The model under review builds one solid part; all positions refer to its coordinate system, in mm. A direction names the side the tool comes from. Coordinates: 2 decimals unless noted, no trailing zeros. Write each loop counter-clockwise with the first axis right and the second up, starting at its lowest first coordinate (ties: lowest second). Pieces come first, ordered by that corner, then holes. Notation, with made-up numbers: (-18.5, 6.5) - (38.5, 6.5) arc R11 ccw to (38.5, 10.5) - close; hole circle Ø10 at (10, 47.25). An arc over 180 degrees is marked (long way). Put each result on its own line as item: value.
from build123d import *

# Parameters (mm, degrees)
SKETCH_2_R          = 2.1
CUT_EXTRUDE_1_DEPTH = 50.216460661
CHAMFER_1_SIZE      = 0.5
CHAMFER_2_SIZE      = 0.5


with BuildPart() as part:
    # Эскиз1 → Повернуть1 (revolve)
    with BuildSketch(Plane.XY, mode=Mode.PRIVATE) as revolve_1_sk:
        Polygon((-22.5, 5), (-22.5, 2), (-20.5, 0), (-15.5, 0), (-15.5, 1.5), (-17.5, 1.5), (-17.5, 19.5), (-18.5, 19.5), (-18.5, 21.1), (-17.5, 21.1), (-17.5, 22.6), (-20, 22.6), (-21, 21.6), (-21, 13), (-32.5, 13), (-32.5, 5), align=None)
    revolve(revolve_1_sk.sketch.rotate(Axis((0, 0, 0), (0, 1, 0)), 270), axis=Axis((0, 0, 0), (0, 1, 0)))

    # Эскиз2 → Вырез-Вытянуть1 (cut, through all)
    with BuildSketch(Plane.XZ.offset(-5)):
        with Locations((0, 27.5)):
            Circle(SKETCH_2_R)
        with Locations((27.5, 0)):
            Circle(SKETCH_2_R)
        with Locations((0, -27.5)):
            Circle(SKETCH_2_R)
        with Locations((-27.5, 0)):
            Circle(SKETCH_2_R)
    extrude(amount=-CUT_EXTRUDE_1_DEPTH, mode=Mode.SUBTRACT)

    # Фаска1
    chamfer_1_edges = [part.edges().sort_by_distance(p)[0] for p in [
        (0, 0, 15.5),
        (0, 1.5, 15.5),
        (0, 22.6, 17.5),
    ]]
    chamfer(chamfer_1_edges, length=CHAMFER_1_SIZE)

    # Фаска2
    chamfer_2_edges = [part.edges().sort_by_distance(p)[0] for p in [
        (-2.1, 13, 27.5),
        (-2.1, 5, 27.5),
        (25.4, 13, 0),
        (25.4, 5, 0),
        (-2.1, 13, -27.5),
        (-2.1, 5, -27.5),
        (-29.6, 13, 0),
        (-29.6, 5, 0),
    ]]
    chamfer(chamfer_2_edges, length=CHAMFER_2_SIZE)


solid = part.part
1. The part is to be moulded in two halves that separate along X. For faces 1 (the cylindrical face through (8.618, 3.479, -20.784)), 2 (the flat face through (11, 0, -12)), 3 (the flat face through (14.2, 1.5, 7.7)), say which applies: +X half, -X half, draft (parallel to the pull), parting line (faces both ways), or undercut.
Determined:
face 1: parting line
face 2: draft
face 3: undercut
2. Consider section C-C on x = 0. Give the number of separate pieces and of enclosed holes in the cut face, plus the area to 3 significant figures.
Determined:
separate pieces: 4
enclosed holes: 0
area: 286 mm^2
3. To check wall thickness, follow probe 1 along X at (y, z) = (21.55, 0); probe 2 along Z at (x, y) = (-0.5, 5.5); probe 3 along Y at (x, z) = (9.5, 21.5). State the ranges of each line that lie inside material, in increasing order.
Determined:
probe 1: x = -21 to -17.5, 17.5 to 21
probe 2: z = -32.5 to -29.54, -25.46 to -17.49, 17.49 to 25.46, 29.54 to 32.5
probe 3: y = 5 to 13
4. Machinability: for faces 4 (the cylindrical face through (1.13, 8.95, -25.73)), 5 (the flat face through (14, 21.1, 11)), 6 (the flat face through (-22, 5, -7)), which of the approach directions +Z, -Z, +X, -X, +Y, -Y give a long, thin tool a straight path to every point of the face, cutting with its end or side? Answer none if there is none.
Determined:
face 4: +Y, -Y
face 5: none
face 6: -Y
5. Consider section D-D on x = -27.5. State the section outline as (y, z) points, plus the area to 3 significant figures.
Determined:
outline: (5, -17.32) - (13, -17.32) - (13, -2.6) - (12.5, -2.1) - (5.5, -2.1) - (5, -2.6) - close; (5, 2.6) - (5.5, 2.1) - (12.5, 2.1) - (13, 2.6) - (13, 17.32) - (5, 17.32) - close
area: 243 mm^2
6. Consider section A-A on y = 10.25. State the section outline as (x, z) points.
Determined:
outline: circle Ø65 at (0, 0); hole circle Ø4.2 at (-27.5, 0); hole circle Ø35 at (0, 0); hole circle Ø4.2 at (0, -27.5); hole circle Ø4.2 at (0, 27.5); hole circle Ø4.2 at (27.5, 0)
7. Consider section B-B on z = 27.5. State the section outline as (x, y) points, plus the area to 3 significant figures.
Determined:
outline: (-17.32, 5) - (-2.6, 5) - (-2.1, 5.5) - (-2.1, 12.5) - (-2.6, 13) - (-17.32, 13) - close; (2.1, 5.5) - (2.6, 5) - (17.32, 5) - (17.32, 13) - (2.6, 13) - (2.1, 12.5) - close
area: 243 mm^2
8. For pin 1 Ø6 at (x, z) = (7.5, -14.5) entering from +Y; pin 2 Ø10 at (y, z) = (7, -25) entering from -X; pin 3 Ø5 at (x, z) = (0, -27.5) entering from +Y; pin 4 Ø4 at (y, z) = (7.5, -7) entering from -X, all flat-tipped, find the tip position at first contact; note any pin that passes through.
Determined:
pin 1: stops at y = 22.6
pin 2: stops at x = -25.62
pin 3: stops at y = 12.9
pin 4: stops at x = -32.11
